Part model, mm, in its own coordinate system. A direction names the side the tool comes from. Round coordinates to 2 decimals unless told otherwise and drop trailing zeros. Loops run counter-clockwise (first coordinate to the right, second up) from the corner with the lowest first, then second, coordinate; pieces in that order, holes last. Notation, with made-up numbers: M 18,11.25 L 41,11.25 A11 cw 41,20.25 Z; hole C 31.5,21 d5. An arc over 180 degrees is marked long. Write each question's results on one line, items separated by ' | '.
from build123d import *

# Parameters (mm, degrees)
SKETCH1_W                                      = 8.5
SKETCH1_H                                      = 8.5
EXTRUDE1_DEPTH                                 = 2.75
SKETCH8_W                                      = 7.8
SKETCH8_H                                      = 7.8
EXTRUDE6_DEPTH                                 = 0.5
SKETCH3_W                                      = 4
SKETCH3_H                                      = 2.75
EXTRUDE3_DEPTH                                 = 3.25
CBORE_FOR_0_SOCKET_HEAD_CAP_SCREW1_D           = 1.778
CBORE_FOR_0_SOCKET_HEAD_CAP_SCREW1_CBORE_D     = 3.175
CBORE_FOR_0_SOCKET_HEAD_CAP_SCREW1_CBORE_DEPTH = 1.524
FILLET1_R                                      = 1


with BuildPart() as part:
    # Sketch1 → Extrude1 (new body)
    with BuildSketch(Plane(origin=(0, 0, 0), x_dir=(1, 0, 0), z_dir=(0, 1, 0))):
        Rectangle(SKETCH1_W, SKETCH1_H)
    extrude(amount=EXTRUDE1_DEPTH)

    # Sketch8 → Extrude6 (cut)
    with BuildSketch(Plane.XZ):
        Rectangle(SKETCH8_W, SKETCH8_H)
    extrude(amount=-EXTRUDE6_DEPTH, mode=Mode.SUBTRACT)

    # Sketch3 → Extrude3 (add)
    with BuildSketch(Plane.XY.offset(4.25)):
        with Locations((-2.25, 1.375)):
            Rectangle(SKETCH3_W, SKETCH3_H)
    extrude(amount=EXTRUDE3_DEPTH)

    # CBORE for #0 Socket Head Cap Screw1 (through all)
    with Locations(Plane(origin=(-2.25, 2.75, 5.5), x_dir=(0, 0, 1), z_dir=(0, 1, 0))):
        with Locations((0, 0)):
            CounterBoreHole(CBORE_FOR_0_SOCKET_HEAD_CAP_SCREW1_D / 2, CBORE_FOR_0_SOCKET_HEAD_CAP_SCREW1_CBORE_D / 2, CBORE_FOR_0_SOCKET_HEAD_CAP_SCREW1_CBORE_DEPTH)

    # Fillet1
    fillet1_edges = [part.edges().sort_by_distance(p)[0] for p in [
        (-3.9, 0.25, 3.9),
        (-3.9, 0.25, -3.9),
        (3.9, 0.25, -3.9),
        (3.9, 0.25, 3.9),
        (-4.25, 1.375, -4.25),
        (4.25, 1.375, -4.25),
        (-0.25, 1.375, 4.25),
        (4.25, 1.375, 4.25),
        (-0.25, 1.375, 7.5),
        (-4.25, 1.375, 7.5),
    ]]
    fillet(fillet1_edges, radius=FILLET1_R)


solid = part.part
Item 1: Which spindle directions (+Z, -Z, +X, -X, +Y, -Y) get a long thin tool onto all of the face, cutting with end or side? Do faces 4 (the cylindrical face through (3.599, 0.254, -3.615)), 5 (the flat face through (2, 1, 4.25)), 6 (the flat face through (-2.23, 1.226, 6.54)). Say none if no direction does.
Filled sheet:
face 4: -Y | face 5: +Z, +X, +Y, -Y | face 6: +Y
Item 2: Wall check: L1, parallel to X at y = 2.15, z = 5.5; L2, parallel to Z at x = -2, y = 0.2; L3, parallel to Y at x = 2, z = 1.5. Give the ranges that are in metal, low to high.
Filled sheet:
L1: -4.25 to -3.84, -0.66 to -0.25 | L2: -4.25 to -3.9, 3.9 to 4.65, 6.35 to 7.5 | L3: 0.5 to 2.75
Item 3: Drop flat-ended pins along their axis: P1, Ø0.6, axis at x = 1, y = 0.5, coming from the +Z side; P2, Ø1.4, axis at y = 1.5, z = 6, coming from the +X side. Give the stop position or say it passes through.
Filled sheet:
P1: z = 4.25 | P2: x = -0.25
Item 4: Two-plate mould, pull along X, no slides. Class faces 1 (the flat face through (0, 2.75, 0)), 2 (the cylindrical face through (-3.615, 0.254, 3.599)), 3 (the flat face through (-0.25, 1, 6)): +X half, -X half, draft (parallel to the pull), parting line (faces both ways), or undercut.
Filled sheet:
face 1: draft | face 2: undercut | face 3: +X half
Item 5: Band-saw the part on B-B on x = -2.25. Give the cut face in (y, z).
Filled sheet:
outline: M 0,-4.25 L 2.75,-4.25 L 2.75,3.91 L 1.23,3.91 L 1.23,4.61 L 0,4.61 L 0,3.9 L 0.5,3.9 L 0.5,-3.9 L 0,-3.9 Z; M 0,6.39 L 1.23,6.39 L 1.23,7.09 L 2.75,7.09 L 2.75,7.5 L 0,7.5 Z
Item 6: Band-saw the part on A-A on z = 5.5. Give the cut face in (x, y), and give its area (3 significant figures).
Filled sheet:
outline: M -4.25,0 L -3.14,0 L -3.14,1.23 L -3.84,1.23 L -3.84,2.75 L -4.25,2.75 Z; M -1.36,0 L -0.25,0 L -0.25,2.75 L -0.66,2.75 L -0.66,1.23 L -1.36,1.23 Z | area: 3.98 mm^2
Item 7: Band-saw the part on C-C on y = 0.9. Give the cut face in (x, z), and give its area (3 significant figures).
Filled sheet:
outline: M -4.25,-3.25 A1 ccw -3.25,-4.25 L 3.25,-4.25 A1 ccw 4.25,-3.25 L 4.25,3.25 A1 ccw 3.25,4.25 L 0.75,4.25 A1 cw -0.25,5.25 L -0.25,6.5 A1 ccw -1.25,7.5 L -3.25,7.5 A1 ccw -4.25,6.5 Z; hole C -2.25,5.5 d1.78 | area: 81.9 mm^2
Item 8: Band-saw the part on D-D on z = 1. Give the cut face in (x, y).
Filled sheet:
outline: M -4.25,0 L -3.9,0 L -3.9,0.5 L 3.9,0.5 L 3.9,0 L 4.25,0 L 4.25,2.75 L -4.25,2.75 Z
